```python
from build123d import *

# Parameters (mm, degrees)
SKETCH1_R            = 4.22275
BOSS_EXTRUDE1_DEPTH  = 3.048
FILLET1_R            = 12.7
CUT_EXTRUDE1_DEPTH   = 120.852046006
FILLET2_R            = 5.08
FILLET2_OF_MIRROR1_R = 5.08
BOSS_EXTRUDE2_DEPTH  = 3.048
FILLET4_R            = 6.35


with BuildPart() as part:
    # Sketch1 → Boss-Extrude1 (new body)
    with BuildSketch(Plane.XY):
        with BuildLine():
            Line((51.054, 0), (-51.054, 0))
            Line((-51.054, 0), (-51.054, -3.048))
            Line((-51.054, -3.048), (-63.754, -3.048))
            Line((-63.754, -3.048), (-63.754, 0))
            Line((-63.754, 0), (-94.861600757, 0))
            ThreePointArc((-94.861600757, 0), (-96.657651981, 0.743948776), (-97.401600757, 2.54))
            Line((-97.401600757, 2.54), (-97.401600757, 22.606))
            Line((-97.401600757, 22.606), (-100.449600757, 22.606))
            Line((-100.449600757, 22.606), (-100.449600757, 35.306))
            Line((-100.449600757, 35.306), (-97.401600757, 35.306))
            Line((-97.401600757, 35.306), (-65.034740931, 62.09905242))
            ThreePointArc((-65.034740931, 62.09905242), (-55.791114337, 65.303706753), (-46.712023238, 61.658909525))
            Line((-46.712023238, 61.658909525), (0, 19.05))
            Line((0, 19.05), (46.712023238, 61.658909525))
            ThreePointArc((46.712023238, 61.658909525), (55.791114337, 65.303706753), (65.034740931, 62.09905242))
            Line((65.034740931, 62.09905242), (97.401600757, 35.306))
            Line((97.401600757, 35.306), (100.449600757, 35.306))
            Line((100.449600757, 35.306), (100.449600757, 22.606))
            Line((100.449600757, 22.606), (97.401600757, 22.606))
            Line((97.401600757, 22.606), (97.401600757, 2.54))
            ThreePointArc((97.401600757, 2.54), (96.657651981, 0.743948776), (94.861600757, 0))
            Line((94.861600757, 0), (63.754, 0))
            Line((63.754, 0), (63.754, -3.048))
            Line((63.754, -3.048), (51.054, -3.048))
            Line((51.054, -3.048), (51.054, 0))
        make_face()
        with Locations((56.126600757, 51.33773565)):
            Circle(SKETCH1_R, mode=Mode.SUBTRACT)
        with Locations((-56.126600757, 51.33773565)):
            Circle(SKETCH1_R, mode=Mode.SUBTRACT)
    extrude(amount=-BOSS_EXTRUDE1_DEPTH)

    # Fillet1
    fillet1_edges = [part.edges().sort_by_distance(p)[0] for p in [
        (0, 19.05, -1.524),
    ]]
    fillet(fillet1_edges, radius=FILLET1_R)

    # Sketch3 → Cut-Extrude1 (cut, symmetric)
    with BuildSketch(Plane.XY):
        with BuildLine():
            Line((-64.628984538, 37.704829039), (-78.351600757, 26.345346603))
            Line((-78.351600757, 26.345346603), (-78.351600757, 7.62))
            Line((-78.351600757, 7.62), (-23.782503148, 7.62))
            Line((-23.782503148, 7.62), (-23.782503148, 15.24))
            Line((-23.782503148, 15.24), (-47.971968454, 37.304699134))
            ThreePointArc((-47.971968454, 37.304699134), (-56.225687634, 40.61815116), (-64.628984538, 37.704829039))
        make_face()
    cut_extrude1 = extrude(amount=CUT_EXTRUDE1_DEPTH, both=True, mode=Mode.SUBTRACT)

    # Fillet2
    fillet2_edges = [part.edges().sort_by_distance(p)[0] for p in [
        (-23.782503148, 15.24, -1.524),
        (-23.782503148, 7.62, -1.524),
        (-78.351600757, 7.62, -1.524),
        (-78.351600757, 26.345346603, -1.524),
    ]]
    fillet(fillet2_edges, radius=FILLET2_R)

    # Mirror1: Cut-Extrude1 across plane
    add(cut_extrude1.mirror(Plane(origin=(0, 0, 0), x_dir=(0, 0, 1), z_dir=(1, 0, 0))), mode=Mode.SUBTRACT)

    # Fillet2 of Mirror1
    fillet2_of_mirror1_edges = [part.edges().sort_by_distance(p)[0] for p in [
        (23.782503148, 15.24, -1.524),
        (23.782503148, 7.62, -1.524),
        (78.351600757, 7.62, -1.524),
        (78.351600757, 26.345346603, -1.524),
    ]]
    fillet(fillet2_of_mirror1_edges, radius=FILLET2_OF_MIRROR1_R)

    # Sketch4 → Boss-Extrude2 (add)
    with BuildSketch(Plane.XY):
        Polygon((-97.401600757, 75.714336407), (-77.552967075, 51.736555375), (-83.791225568, 46.572570123), (-97.401600757, 63.014336407), (-100.449600757, 63.014336407), (-100.449600757, 75.714336407), align=None)
    boss_extrude2 = extrude(amount=-BOSS_EXTRUDE2_DEPTH)

    # Mirror3: Boss-Extrude2 across plane
    add(boss_extrude2.mirror(Plane(origin=(0, 0, 0), x_dir=(0, 0, 1), z_dir=(1, 0, 0))))

    # Fillet4
    fillet4_edges = [part.edges().sort_by_distance(p)[0] for p in [
        (-77.552967075, 51.736555375, -1.524),
        (-83.791225568, 46.572570123, -1.524),
        (77.552967075, 51.736555375, -1.524),
        (83.791225568, 46.572570123, -1.524),
    ]]
    fillet(fillet4_edges, radius=FILLET4_R)


solid = part.part
```
The model under review builds one solid part; all positions refer to its coordinate system, in mm. A direction names the side the tool comes from. Round coordinates to 2 decimals unless told otherwise and drop trailing zeros. Order: outer loops, then holes, each group sorted by start corner. A loop starts at its lowest first (then second) coordinate and runs counter-clockwise, first axis right, second up. Notation, with made-up numbers: (14, 52.5) -> (42, 52.5) arc R26 ccw to (42, 85.5) -> close; hole circle Ø3 at (68.25, -25.5). An arc over 180 degrees is marked (long way). Use a Markdown table: item, result.
Q1. Clearance check with flat-ended pins moving along their axes: P1, Ø1, axis at y = 54, z = -1, coming from the +X side; P2, Ø5, axis at x = 56.13, y = 51.34, coming from the -Z side; P3, Ø1.5, axis at y = 15.5, z = -1.5, coming from the -X side. State where each tip first meets the part, or that it passes through.
Values:
| item | result |
|---|---|
| P1 | stops at x = 90.35 |
| P2 | passes through |
| P3 | stops at x = -97.4 |
Q2. We need section D-D on z = -2.3. State how many separate pieces and enclosed holes the cut face has, then the cut area to 3 significant figures.
Values:
| item | result |
|---|---|
| separate pieces | 1 |
| enclosed holes | 4 |
| area | 7,270 mm^2 |
Q3. Tool access review of faces 1 (the flat face through (27.368, 44.014, -1.503)), 2 (the flat face through (-92.554, 57.158, -1.503)), 3 (the flat face through (92.981, 38.965, -1.503)), 4 (the flat face through (36.548, 26.884, -1.503)): name each direction out of +Z, -Z, +X, -X, +Y, -Y from which nothing blocks a thin tool from reaching the whole face with its end or side.
Values:
| item | result |
|---|---|
| face 1 | +Z, -Z, +Y |
| face 2 | +Z, -Z, -X |
| face 3 | +Z, -Z, +X |
| face 4 | +Z, -Z |
Q4. We need section B-B on y = 71. Write out the cut boundary in (x, z), then the cut area to 3 significant figures.
Values:
| item | result |
|---|---|
| outline | (-100.45, -3.05) -> (-93.5, -3.05) -> (-93.5, 0) -> (-100.45, 0) -> close; (93.5, -3.05) -> (100.45, -3.05) -> (100.45, 0) -> (93.5, 0) -> close |
| area | 42.4 mm^2 |
Q5. We need section A-A on x = -41. Write out the cut boundary in (y, z), then the cut area to 3 significant figures.
Values:
| item | result |
|---|---|
| outline | (0, -3.05) -> (7.62, -3.05) -> (7.62, 0) -> (0, 0) -> close; (30.95, -3.05) -> (56.45, -3.05) -> (56.45, 0) -> (30.95, 0) -> close |
| area | 101 mm^2 |
Q6. We need section C-C on y = 5. Write out the cut boundary in (x, z), then the cut area to 3 significant figures.
Values:
| item | result |
|---|---|
| outline | (-97.4, -3.05) -> (97.4, -3.05) -> (97.4, 0) -> (-97.4, 0) -> close |
| area | 594 mm^2 |
Q7. For line 1 (X direction, y = 13.5, z = -1.5); line 2 (X direction, y = 26, z = -2.3); line 3 (Y direction, x = -53.5, z = -1.25), list the stretches that pass through material, from the lowest coordinate up.
Values:
| item | result |
|---|---|
| line 1 | x = -97.4 to -78.35, -23.81 to 23.81, 78.35 to 97.4 |
| line 2 | x = -100.45 to -77.92, -35.58 to -7.51, 7.51 to 35.58, 77.92 to 100.45 |
| line 3 | y = -3.05 to 7.62, 40.25 to 48.03, 54.64 to 65.06 |
